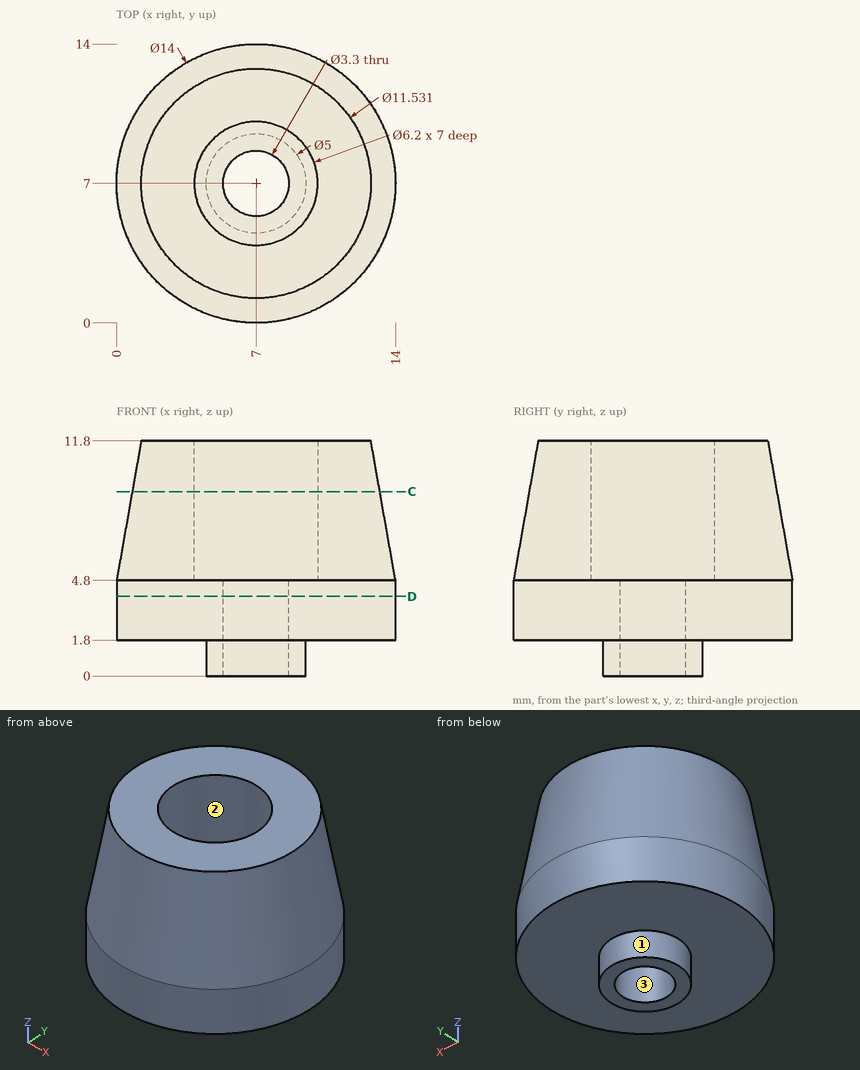
Check sheet for the drawn part. Datum: minimum x, y, z corner. Units: mm. A direction names the side the tool comes from. Give positions to 0.01 mm unless a question says otherwise; leave off trailing zeros. Loops run counter-clockwise (first coordinate to the right, second up) from the corner with the lowest first, then second, coordinate; pieces in that order, holes last. Notation, with made-up numbers: M 1,45 L 17,45 A28 cw 17,66 Z; hole C 19.25,52 d9. An arc over 180 degrees is marked long. Answer as CSV lines item,"result".
Item 1: Scan lines: L1, parallel to Z at x = 12.25, y = 5.5; L2, parallel to Z at x = 9, y = 9; L3, parallel to X at y = 9.75, z = 7.75 (1 decimal). Record each from-to range of solid material in increasing order.
Reply:
L1,"1.8 to 11.8"
L2,"1.8 to 4.8"
L3,"1.1 to 5.6, 8.4 to 12.9"
Item 2: Depth check by flat-ended pin: pin 1 Ø6 at (y, z) = (2.5, 6.5) entering from -X; pin 2 Ø5 at (x, y) = (7, 7) entering from +Z; pin 3 Ø1.5 at (x, z) = (11, 6) entering from -Y. Enter the tip coordinate at first touch or a pass-through.
Reply:
pin 1,"x = 0.3"
pin 2,"z = 4.8"
pin 3,"y = 1.01"
Item 3: Sectioned sample at C-C, the plane z = 9.25. Enter the section's corners in (x, y) (1 decimal).
Reply:
outline,"C 7,7 d12.4; hole C 7,7 d6.2"
Item 4: Set-up check for the marked faces 1, 2 and 3: record each of +Z, -Z, +X, -X, +Y, -Y from which the full face is reachable in a straight line by a thin tool's end or side.
Reply:
face 1,"-Z"
face 2,"+Z"
face 3,"+Z, -Z"
Item 5: Sectioned sample at D-D, the plane z = 4. Enter the section's corners in (x, y), then the cut area to 3 significant figures.
Reply:
outline,"C 7,7 d14; hole C 7,7 d3.3"
area,"145 mm^2"
